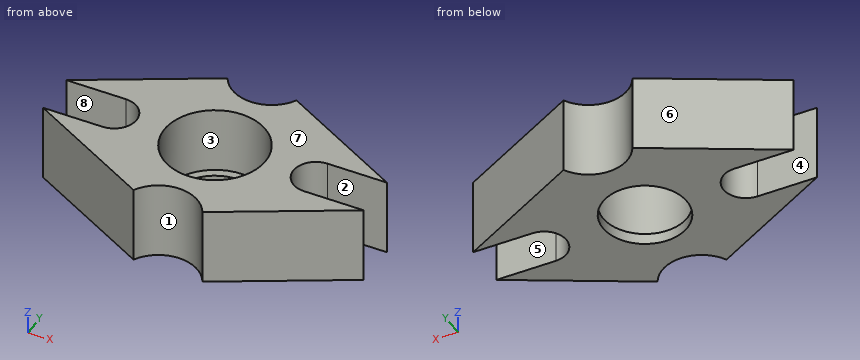
from build123d import *

# Parameters (mm, degrees)
F0_R      = 9
F1_DEPTH  = 12
F1_FACE_R = 9
F0_R_2    = 7.5
F2_DEPTH  = 2


with BuildPart() as f1:
    # F0 (on Top) → F1 (new body)
    with BuildSketch(Plane.XY):
        with BuildLine():
            ThreePointArc((6.155044, 16.166018), (0, 12.5), (-6.155044, 16.166018))
            Line((-6.155044, 16.166018), (-28.615385, 4))
            Line((-28.615385, 4), (-18, 4))
            ThreePointArc((-18, 4), (-14, 0), (-18, -4))
            Line((-18, -4), (-28.615385, -4))
            Line((-28.615385, -4), (-6.155044, -16.166018))
            ThreePointArc((-6.155044, -16.166018), (0, -12.5), (6.155044, -16.166018))
            Line((6.155044, -16.166018), (28.615385, -4))
            Line((28.615385, -4), (18, -4))
            ThreePointArc((18, -4), (14, 0), (18, 4))
            Line((18, 4), (28.615385, 4))
            Line((28.615385, 4), (6.155044, 16.166018))
        make_face()
        Circle(F0_R, mode=Mode.SUBTRACT)
    extrude(amount=F1_DEPTH)

    # F1_face (on face) + F0 (on Top) → F2 (join)
    with BuildSketch(Plane.XY.offset(12)):
        with BuildLine():
            ThreePointArc((-6.155044, -16.166018), (0, -12.5), (6.155044, -16.166018))
            Line((6.155044, -16.166018), (28.615385, -4))
            Line((28.615385, -4), (18, -4))
            ThreePointArc((18, -4), (14, 0), (18, 4))
            Line((18, 4), (28.615385, 4))
            Line((28.615385, 4), (6.155044, 16.166018))
            ThreePointArc((6.155044, 16.166018), (0, 12.5), (-6.155044, 16.166018))
            Line((-6.155044, 16.166018), (-28.615385, 4))
            Line((-28.615385, 4), (-18, 4))
            ThreePointArc((-18, 4), (-14, 0), (-18, -4))
            Line((-18, -4), (-28.615385, -4))
            Line((-28.615385, -4), (-6.155044, -16.166018))
        make_face()
        Circle(F1_FACE_R, mode=Mode.SUBTRACT)
    with BuildSketch(Plane.XY):
        Circle(F0_R)
        Circle(F0_R_2, mode=Mode.SUBTRACT)
    extrude(amount=F2_DEPTH)


solid = f1.part
Read the model definition and answer for the solid it produces. Units are mm, in the model's axes. Face numbers are marked on the shaded views. A direction names the side the tool comes from. Coordinates: 2 decimals unless noted, no trailing zeros. Write each loop counter-clockwise with the first axis right and the second up, starting at its lowest first coordinate (ties: lowest second). Pieces come first, ordered by that corner, then holes. Notation, with made-up numbers: (23.25, -1.75) - (56.25, -1.75) arc R10 ccw to (56.25, 9.25) - close; hole circle Ø5 at (33.5, -33.75). An arc over 180 degrees is marked (long way). One line per question, with ' | ' between items.
Q1. Find section D-D, the plane x = -24. Write down the section's boundary in (y, z), plus the area to 3 significant figures.
Result set:
outline: (-6.5, 0) - (-4, 0) - (-4, 14) - (-6.5, 14) - close; (4, 0) - (6.5, 0) - (6.5, 14) - (4, 14) - close | area: 70.0 mm^2
Q2. Each of these flat-tipped pins is pushed along its axis until it touches: P1, Ø3, axis at x = -1, z = 11, coming from the +Y side; P2, Ø1, axis at x = 16, z = 10.5, coming from the +Y side; P3, Ø6, axis at y = -10.5, z = 6, coming from the -X side; P4, Ø9, axis at x = 4.5, y = -4, coming from the +Z side. Where does it stop, or does it pass through?
Result set:
P1: y = 12.96 | P2: y = 11.1 | P3: x = -22.15 | P4: z = 14
Q3. Consider L1, parallel to X at y = -6, z = 12; L2, parallel to Y at x = -5, z = 12; L3, parallel to Y at x = 2, z = 10.25. Determine where each line is inside the solid, lowest interval first. Write a range as [from, to].
Result set:
L1: [-24.92, -6.71], [6.71, 24.92] | L2: [-14.6, -7.48], [7.48, 14.6] | L3: [-12.79, -8.77], [8.77, 12.79]
Q4. Find section C-C, the plane y = 0. Write down the section's boundary in (x, z).
Result set:
outline: (-14, 0) - (-7.5, 0) - (-7.5, 2) - (-9, 2) - (-9, 14) - (-14, 14) - close; (7.5, 0) - (14, 0) - (14, 14) - (9, 14) - (9, 2) - (7.5, 2) - close
Q5. For the marked faces 1, 2, 3 and 4, determine the directions among +Z, -Z, +X, -X, +Y, -Y from which every point of the face is accessible in a straight line to the end or side of a thin tool.
Result set:
face 1: +Z, -Z, -Y | face 2: +Z, -Z, +X | face 3: +Z | face 4: +Z, -Z, -X
Q6. Determine the mould class of the marked faces 5, 6, 7 and 8 for opening direction Y: +Y half, -Y half, draft (parallel to the pull), parting line (faces both ways), or undercut.
Result set:
face 5: undercut | face 6: +Y half | face 7: draft | face 8: undercut
Q7. Find section A-A, the plane z = 4. Write down the section's boundary in (x, y).
Result set:
outline: (-28.62, -4) - (-6.16, -16.17) arc R7 cw to (6.16, -16.17) - (28.62, -4) - (18, -4) arc R4 cw to (18, 4) - (28.62, 4) - (6.16, 16.17) arc R7 cw to (-6.16, 16.17) - (-28.62, 4) - (-18, 4) arc R4 cw to (-18, -4) - close; hole circle Ø18 at (0, 0)
Q8. Find section B-B, the plane x = 0. Write down the section's boundary in (y, z), plus the area to 3 significant figures.
Result set:
outline: (-12.5, 0) - (-7.5, 0) - (-7.5, 2) - (-9, 2) - (-9, 14) - (-12.5, 14) - close; (7.5, 0) - (12.5, 0) - (12.5, 14) - (9, 14) - (9, 2) - (7.5, 2) - close | area: 104 mm^2
